Can you work these out from the model? Positions are in its coordinate system, mm. Round coordinates to 2 decimals unless told otherwise and drop trailing zeros. Write each loop counter-clockwise with the first axis right and the second up, starting at its lowest first coordinate (ties: lowest second). Pieces come first, ordered by that corner, then holes. Notation, with made-up numbers: (-9.75, 70.5) - (13.25, 70.5) arc R26 cw to (13.25, 96.5) - close; hole circle Ø9 at (-25, 32.5). An arc over 180 degrees is marked (long way). One line per item, written item: value. Start each with the question number.
(1) I want a section at A-A on z = 10. List the corners of the cut face in (x, y) for me.
(2) I want a section at C-C on x = 64. List the corners of the cut face in (y, z) for me.
(3) I want a section at B-B on x = 16. List the corners of the cut face in (y, z) for me, plus the area to 3 significant figures.
(4) I'm going to push flat-ended pins straight in: pin 1 Ø1.2 at (y, z) = (13.5, 5.5) entering from +X; pin 2 Ø0.8 at (y, z) = (-9, 4.5) entering from -X; pin 3 Ø15.5 at (x, y) = (20.02, 5.62) entering from +Z. Where does each tip first touch, or does it pass through?
(5) If I drill on L1, parallel to X at y = 1, z = 2; L2, parallel to Y at x = 77.5, z = 5.75; L3, parallel to X at y = 2, z = 13.5, over which ranges is the centre line in solid material (lowest first)? Write a range as from..to.
from build123d import *

# Parameters (mm, degrees)
F0_W      = 130
F0_H      = 53
F1_DEPTH  = 15
F2_R      = 1.25
F5_DEPTH  = 35
F3_R      = 1.25
F6_DEPTH  = 53
F4_R      = 1.25
F7_DEPTH  = 35
F9_DEPTH  = 15
F10_R     = 9.75
F11_DEPTH = 15


with BuildPart() as f1:
    # F0 (on Top) → F1 (new body)
    with BuildSketch(Plane.XY):
        with Locations((20.023906, 2.124549)):
            Rectangle(F0_W, F0_H)
    extrude(amount=F1_DEPTH)

    # F2 (on face) → F5 (cut)
    with BuildSketch(Plane.YZ.offset(85.023906)):
        with Locations((-9.375451, 5)):
            Circle(F2_R)
        with Locations((13.624549, 5)):
            Circle(F2_R)
    extrude(amount=-F5_DEPTH, mode=Mode.SUBTRACT)

    # F3 (on face) → F6 (cut, through all)
    with BuildSketch(Plane.XZ.offset(24.375451)):
        with Locations((-4.976094, 5)):
            Circle(F3_R)
        with Locations((45.023906, 5)):
            Circle(F3_R)
    extrude(amount=-F6_DEPTH, mode=Mode.SUBTRACT)

    # F4 (on face) → F7 (cut)
    with BuildSketch(Plane(origin=(-44.976094, 0, 0), x_dir=(0, -1, 0), z_dir=(-1, 0, 0))):
        with Locations((-13.624549, 5)):
            Circle(F4_R)
        with Locations((9.375451, 5)):
            Circle(F4_R)
    extrude(amount=-F7_DEPTH, mode=Mode.SUBTRACT)

    # F8 (on face) → F9 (cut, through all)
    with BuildSketch(Plane.XY.offset(15)):
        with BuildLine():
            Line((66.523906, -1.249315), (66.523906, 12.498412))
            ThreePointArc((66.523906, 12.498412), (56.023906, 5.624549), (66.523906, -1.249315))
        make_face()
        with BuildLine():
            ThreePointArc((-26.476094, -1.249315), (-19.368175, -0.650401), (-15.976094, 5.624549))
            ThreePointArc((-15.976094, 5.624549), (-19.368175, 11.899499), (-26.476094, 12.498412))
            Line((-26.476094, 12.498412), (-26.476094, -1.249315))
        make_face()
    extrude(amount=-F9_DEPTH, mode=Mode.SUBTRACT)

    # F10 (on face) → F11 (cut, through all)
    with BuildSketch(Plane.XY.offset(15)):
        with Locations((20.023906, 5.624549)):
            Circle(F10_R)
    extrude(amount=-F11_DEPTH, mode=Mode.SUBTRACT)


solid = f1.part
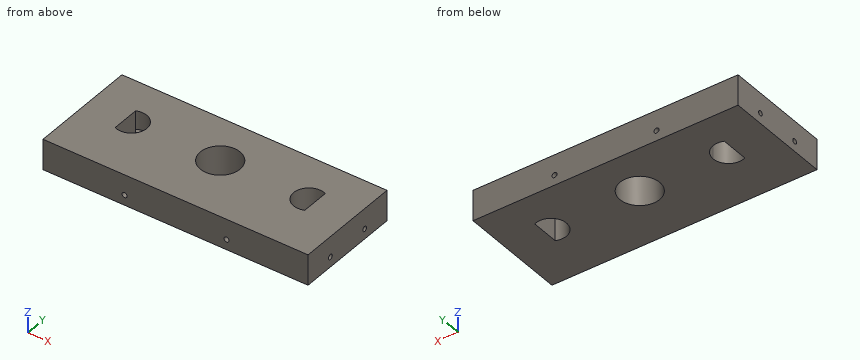
Established:
1. outline: (-44.98, -24.38) - (85.02, -24.38) - (85.02, 28.62) - (-44.98, 28.62) - close; hole (-26.48, -1.25) arc R7.5 ccw to (-15.98, 5.62) arc R7.5 ccw to (-26.48, 12.5) - close; hole circle Ø19.5 at (20.02, 5.62); hole (66.52, -1.25) - (66.52, 12.5) arc R7.5 ccw (long way) to start
2. outline: (-24.38, 0) - (-1.86, 0) - (-1.86, 15) - (-24.38, 15) - close; (13.11, 0) - (28.62, 0) - (28.62, 15) - (13.11, 15) - (13.11, 6.14) arc R1.25 cw (long way) to (13.11, 3.86) - close; hole circle Ø2.5 at (-9.38, 5)
3. outline: (-24.38, 0) - (-3.26, 0) - (-3.26, 15) - (-24.38, 15) - close; (14.51, 0) - (28.62, 0) - (28.62, 15) - (14.51, 15) - close
3. area: 529 mm2
4. pin 1: x = 50.02
4. pin 2: x = -9.98
4. pin 3: through
5. L1: -44.98..-26.48, -17.57..11.44, 28.61..57.62, 66.52..85.02
5. L2: -24.38..-10.38, -8.38..12.62, 14.62..28.62
5. L3: -44.98..-26.48, -16.91..10.97, 29.08..56.96, 66.52..85.02
